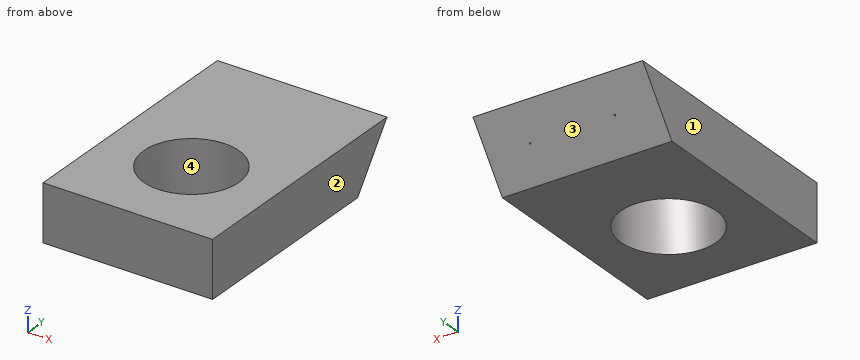
Autodesk Inventor part; units mm, degrees
ref_plane "YZ Plane" through (0, 0, 0) normal (1, 0, 0) x (0, 1, 0)
ref_plane "XZ Plane" through (0, 0, 0) normal (0, 1, 0) x (-1, 0, 0)
ref_plane "XY Plane" through (0, 0, 0) normal (0, 0, 1) x (1, 0, 0)
sketch "Sketch1" plane through (0, 0, 0) normal (1, 0, 0) x (0, 1, 0)
  line L0 (0, 0) -> (170, 0)
  line L1 (0, 0) -> (0, -38)
  line L2 (170, 0) -> (141.3649, -38)
  line L3 (170, 0) -> (170.6921, 0) construction
  line L4 (0, -38) -> (141.3649, -38)
  dimension "d2" = 170
  dimension "d4" = 38
  dimension "d26" = 127
extrude "Extrusion1" add sketch "Sketch1" along normal blind 114
sketch "Sketch4" plane through (0, 170, 0) normal (0, 0.7986, -0.6018) x (1, 0, 0)
  line L0 (0, 47.5812) -> (114, 47.5812)
  circle A0 centre (85.5, 23.7906) radius 2.921
  line L1 (0, 0) -> (0, 47.5812)
  line L2 (0, 0) -> (114, 0)
  line L3 (85.5, 23.7906) -> (28.5, 23.7906) construction
  line L4 (57, 47.5812) -> (57, 0) construction
  point P0 (0, 102.3086)
  point P1 (57, 23.7906)
  dimension "d30" = 57
  dimension "d42" = 28.5
hole "Hole2" at (28.5, 155.6825, -19) at (85.5, 155.6825, -19) direction (0, -0.7986, 0.6018) diameter 1 depth 25.4 tip angle 118
sketch "Sketch5" plane through (0, 0, 0) normal (0, 0, 1) x (1, 0, 0)
  line L0 (0, 170) -> (114, 170)
  circle A0 centre (57, 62) radius 32
  dimension "d44" = 64
  dimension "d45" = 108
hole "Hole3" at (57, 62, 0) direction (0, 0, -1) diameter 64 end through all
properties part number "2p4irsh" material "Wood (Cherry)"
Design review of the part built by this model. Coordinates are the model's own, in mm. Face numbers are marked on the shaded views. Round coordinates to 2 decimals unless told otherwise and drop trailing zeros. Write each loop counter-clockwise with the first axis right and the second up, starting at its lowest first coordinate (ties: lowest second). Pieces come first, ordered by that corner, then holes.
Item 1: We need section D-D on x = 15. Write out the cut boundary in (y, z), and give its area (3 significant figures).
Item 2: The part is to be moulded in two halves that separate along X. For the marked faces 1, 2, 3 and 4, say which applies: +X half, -X half, draft (parallel to the pull), parting line (faces both ways), or undercut.
Item 3: Clearance check with flat-ended pins moving along their axes: pin 1 Ø4 at (x, z) = (62.5, -20.5) entering from +Y; pin 2 Ø10 at (x, z) = (86, -25.5) entering from +Y; pin 3 Ø4 at (x, z) = (92, -19) entering from +Y. State where each tip first meets the part, or that it passes through.
Item 4: We need section B-B on x = 57. Write out the cut boundary in (y, z), and give its area (3 significant figures).
Item 5: For probe 1 along X at (y, z) = (62, -23); probe 2 along Y at (x, z) = (40.5, -31); probe 3 along X at (y, z) = (74.5, -12.5), list the stretches that pass through material, from the lowest coordinate up.
Item 6: We need section A-A on y = 62. Write out the cut boundary in (x, z).
Item 7: We need section C-C on z = -28. Write out the cut boundary in (x, y), and give its area (3 significant figures).
Returned:
1. outline: (0, -38) - (141.36, -38) - (170, 0) - (0, 0) - close
1. area: 5,920 mm2
2. face 1: -X half
2. face 2: +X half
2. face 3: draft
2. face 4: undercut
3. pin 1: stops at y = 156.06
3. pin 2: stops at y = 154.55
3. pin 3: stops at y = 157.19
4. outline: (0, -38) - (30, -38) - (30, 0) - (0, 0) - close; (94, -38) - (141.36, -38) - (170, 0) - (94, 0) - close
4. area: 3,480 mm2
5. probe 1: x = 0 to 25, 89 to 114
5. probe 2: y = 0 to 34.58, 89.42 to 146.64
5. probe 3: x = 0 to 27.54, 86.46 to 114
6. outline: (0, -38) - (25, -38) - (25, 0) - (0, 0) - close; (89, -38) - (114, -38) - (114, 0) - (89, 0) - close
7. outline: (0, 0) - (114, 0) - (114, 148.9) - (0, 148.9) - close; hole circle Ø64 at (57, 62)
7. area: 13,800 mm2
